from build123d import *

# Parameters (mm, degrees)
F0_W     = 109.22
F0_H     = 38.1
F0_R     = 2.4257
F0_R_2   = 2.0193
F1_DEPTH = 3.175


with BuildPart() as f1:
    # F0 (on Top) → F1 (new body)
    with BuildSketch(Plane.XY):
        Rectangle(F0_W, F0_H)
        with Locations((-48.26, -12.7)):
            Circle(F0_R, mode=Mode.SUBTRACT)
        with Locations((48.26, -12.7)):
            Circle(F0_R, mode=Mode.SUBTRACT)
        with Locations((-18, 6.6548)):
            Circle(F0_R_2, mode=Mode.SUBTRACT)
        with Locations((-48.26, 12.7)):
            Circle(F0_R, mode=Mode.SUBTRACT)
        with Locations((18, 6.6548)):
            Circle(F0_R_2, mode=Mode.SUBTRACT)
        with Locations((48.26, 12.7)):
            Circle(F0_R, mode=Mode.SUBTRACT)
    extrude(amount=F1_DEPTH)


solid = f1.part
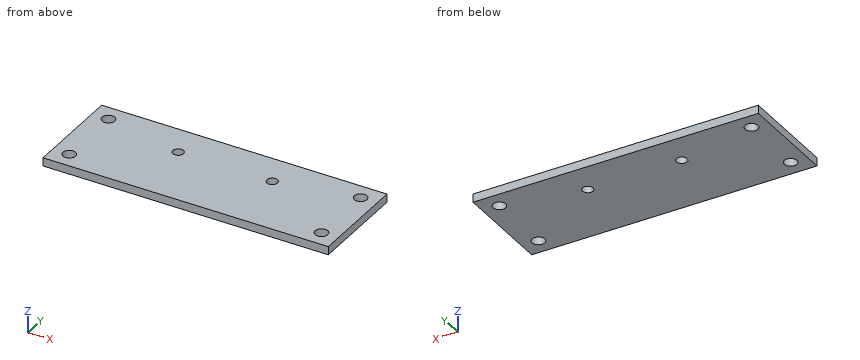
The model under review builds one solid part; all positions refer to its coordinate system, in mm. Round coordinates to 2 decimals unless told otherwise and drop trailing zeros. Write each loop counter-clockwise with the first axis right and the second up, starting at its lowest first coordinate (ties: lowest second). Pieces come first, ordered by that corner, then holes. Notation, with made-up numbers: M 83.25,8.5 L 104.25,8.5 A26 cw 104.25,31.5 Z; hole C -37,78 d2. An arc over 180 degrees is marked long. Answer as CSV lines item,"result". Start each with the question number.
Q1. Consider section C-C, the plane x = -48.26. Give the boundary of the cut face in (y, z) (3 decimals).
Q2. Wall thickness on line 1 along Y through (x, z) = (48.26, 2); line 2 along X through (y, z) = (-13, 1.4); line 3 along Y through (x, z) = (46.5, 0.25): over which ranges is each line inside the solid? List them lowest first.
Q3. Consider section B-B, the plane y = -12.7. Give the boundary of the cut face in (x, z) (3 decimals).
Q4. Consider section D-D, the plane z = 1.4. Give the boundary of the cut face in (x, y), then the cut area to 3 significant figures.
Result set:
1,outline,"M -19.05,0 L -15.126,0 L -15.126,3.175 L -19.05,3.175 Z; M -10.274,0 L 10.274,0 L 10.274,3.175 L -10.274,3.175 Z; M 15.126,0 L 19.05,0 L 19.05,3.175 L 15.126,3.175 Z"
2,line 1,"y = -19.05 to -15.13, -10.27 to 10.27, 15.13 to 19.05"
2,line 2,"x = -54.61 to -50.67, -45.85 to 45.85, 50.67 to 54.61"
2,line 3,"y = -19.05 to -14.37, -11.03 to 11.03, 14.37 to 19.05"
3,outline,"M -54.61,0 L -50.686,0 L -50.686,3.175 L -54.61,3.175 Z; M -45.834,0 L 45.834,0 L 45.834,3.175 L -45.834,3.175 Z; M 50.686,0 L 54.61,0 L 54.61,3.175 L 50.686,3.175 Z"
4,outline,"M -54.61,-19.05 L 54.61,-19.05 L 54.61,19.05 L -54.61,19.05 Z; hole C -48.26,-12.7 d4.85; hole C -48.26,12.7 d4.85; hole C -18,6.65 d4.04; hole C 18,6.65 d4.04; hole C 48.26,-12.7 d4.85; hole C 48.26,12.7 d4.85"
4,area,"4,060 mm²"
